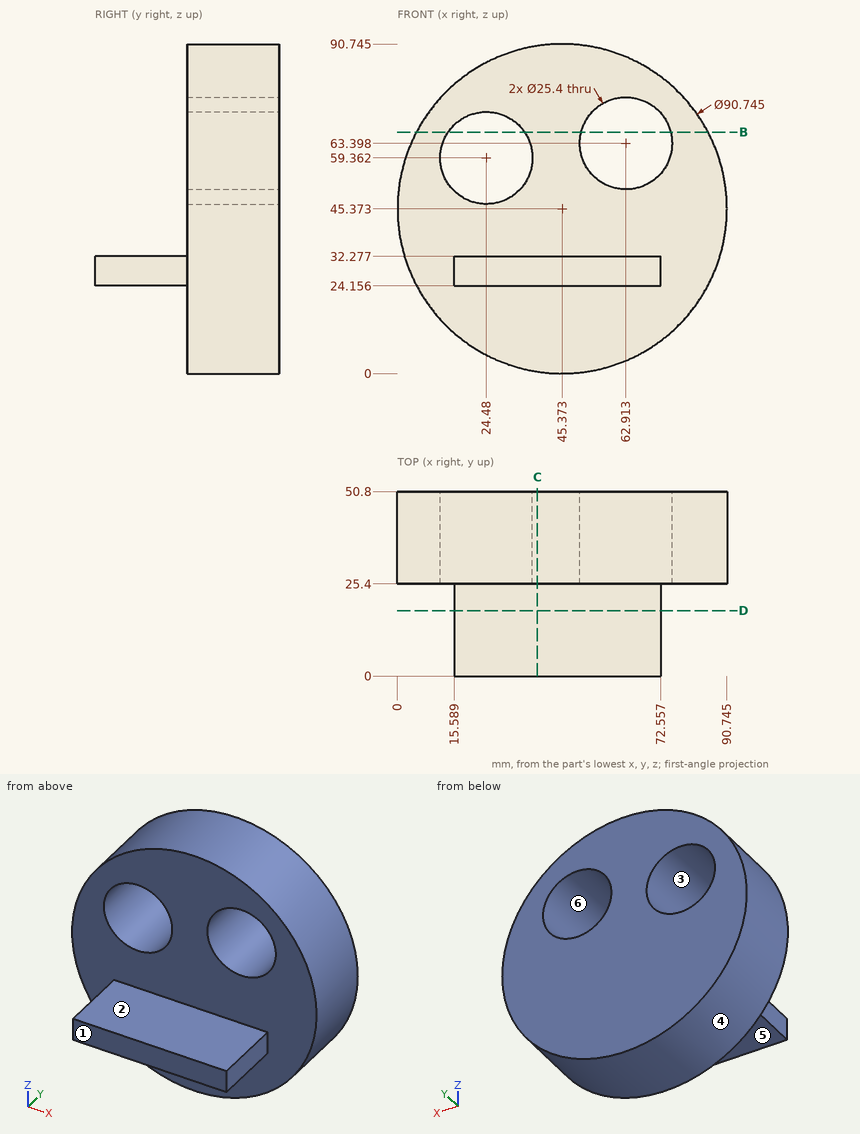
Answer from the drawing. Dimensions are ordinates in mm from the lowest x, y and z of the part. A direction names the side the tool comes from. Give positions to 0.01 mm unless a question says otherwise; leave off trailing zeros. Order: outer loops, then holes, each group sorted by start corner. A loop starts at its lowest first (then second) coordinate and runs counter-clockwise, first axis right, second up. Notation, with made-up numbers: (-36, 52) - (-13, 52) arc R15 ccw to (-13, 75) - close; hole circle Ø2 at (51, 21.5). An arc over 180 degrees is marked (long way). One line per item, written item: value. Start each with the question number.
1. Consider line 1 (Y direction, x = 42, z = 62); line 2 (Z direction, x = 52, y = 22); line 3 (X direction, y = 46.5, z = 53) (1 decimal). Determine where each line is inside the solid, lowest interval first.
2. Section D-D, the plane y = 18 is taken. Write down the section's boundary in (x, z), then the cut area to 3 significant figures.
3. For a pull along X with two mould halves and no side action, classify the marked faces 3, 4, 5 and 6 as released by +X, released by -X, zero draft, split by the parting line, or undercut.
4. Section C-C, the plane x = 38.5 is taken. Write down the section's boundary in (y, z), then the cut area to 3 significant figures.
5. Which of the six approach directions +Z, -Z, +X, -X, +Y, -Y give full straight-line access (tool end or side, diameter ignored) to the marked faces 1 and 2?
6. Each of these flat-tipped pins is pushed along its axis until it touches: pin 1 Ø9 at (y, z) = (9.5, 29) entering from +X; pin 2 Ø20.5 at (x, y) = (32.5, 12.5) entering from -Z; pin 3 Ø10 at (x, y) = (11, 6.5) entering from +Z. Where does it stop, or does it pass through?
7. Section B-B, the plane z = 66.5 is taken. Write down the section's boundary in (x, y) (1 decimal).
Filled sheet:
1. line 1: 25.4 to 50.8
1. line 2: 24.16 to 32.28
1. line 3: 0.6 to 13.5, 35.5 to 55.6, 70.2 to 90.1
2. outline: (15.59, 24.16) - (72.56, 24.16) - (72.56, 32.28) - (15.59, 32.28) - close
2. area: 463 mm²
3. face 3: undercut
3. face 4: split by the parting line
3. face 5: zero draft
3. face 6: undercut
4. outline: (0, 24.16) - (25.4, 24.16) - (25.4, 0.52) - (50.8, 0.52) - (50.8, 90.22) - (25.4, 90.22) - (25.4, 32.28) - (0, 32.28) - close
4. area: 2,480 mm²
5. face 1: +Z, -Z, +X, -X, -Y
5. face 2: +Z, +X, -X, -Y
6. pin 1: x = 72.56
6. pin 2: z = 24.16
6. pin 3: z = 32.28
7. outline: (5.2, 25.4) - (14, 25.4) - (14, 50.8) - (5.2, 50.8) - close; (35, 25.4) - (50.6, 25.4) - (50.6, 50.8) - (35, 50.8) - close; (75.2, 25.4) - (85.5, 25.4) - (85.5, 50.8) - (75.2, 50.8) - close
